Geometry check sheet. Reference: drawing and pictorial views, mm from the part's lowest x, y, z. A direction names the side the tool comes from. Round coordinates to 2 decimals unless told otherwise and drop trailing zeros. Write each loop counter-clockwise with the first axis right and the second up, starting at its lowest first coordinate (ties: lowest second). Pieces come first, ordered by that corner, then holes. Notation, with made-up numbers: M -11.75,57.25 L 13.25,57.25 A25 ccw 13.25,92.25 Z; hole C 28,-6 d10. An arc over 180 degrees is marked long. Answer in a Markdown table with one row per item.
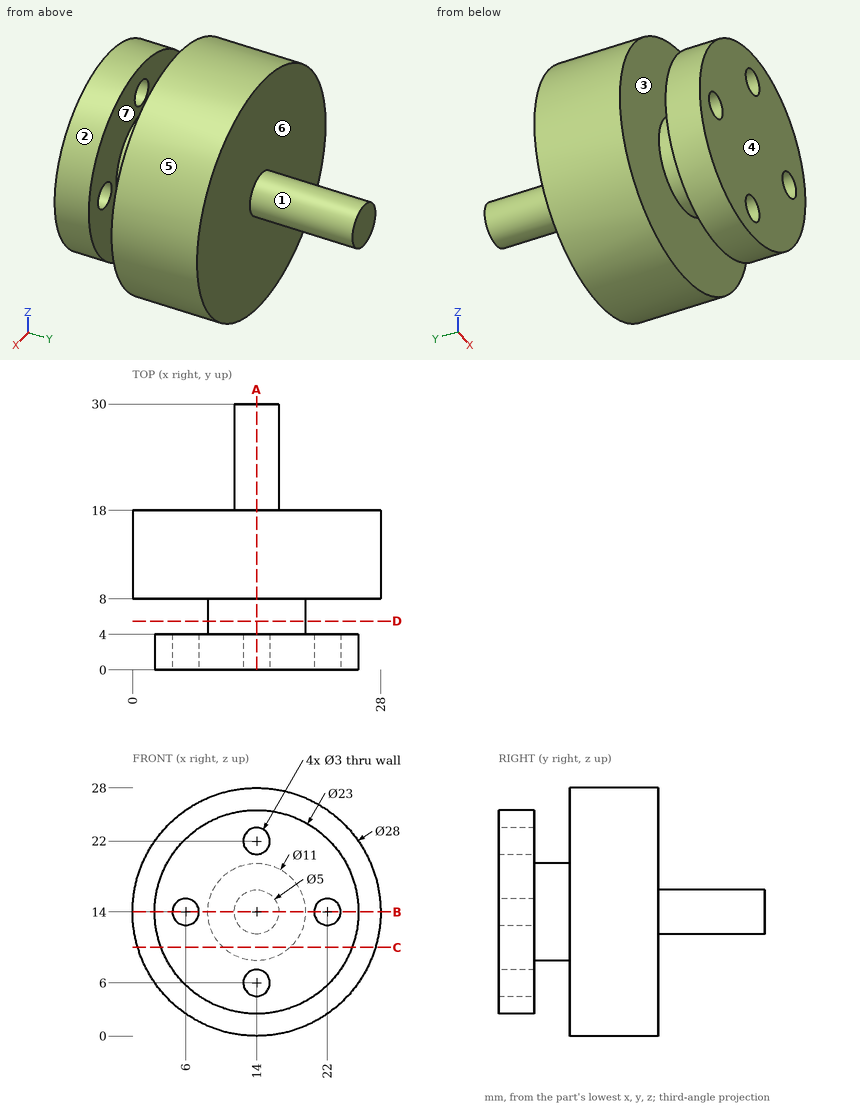
1. Section check C-C, the plane z = 10. Record the cut outline in (x, y).
Found:
| item | result |
|---|---|
| outline | M 0.58,8 L 10.23,8 L 10.23,4 L 3.22,4 L 3.22,0 L 24.78,0 L 24.78,4 L 17.77,4 L 17.77,8 L 27.42,8 L 27.42,18 L 0.58,18 Z |
2. Scan lines: L1, parallel to X at y = 3, z = 14; L2, parallel to Y at x = 8.5, z = 23; L3, parallel to Y at x = 18.5, z = 25.5. Record each from-to range of solid material in increasing order.
Found:
| item | result |
|---|---|
| L1 | x = 2.5 to 4.5, 7.5 to 20.5, 23.5 to 25.5 |
| L2 | y = 0 to 4, 8 to 18 |
| L3 | y = 8 to 18 |
3. Draft check along Y on the marked faces 4, 5, 6 and 7. Enter one of: +Y half, -Y half, draft (parallel to the pull), parting line (faces both ways), or undercut.
Found:
| item | result |
|---|---|
| face 4 | -Y half |
| face 5 | draft |
| face 6 | +Y half |
| face 7 | undercut |
4. Go/stop test with flat-tipped pins: pin 1 (3 mm diameter, centred on y = 5, z = 10, fed in from -X); pin 2 (3 mm diameter, centred on x = 7.5, y = 3.5, fed in from +Z); pin 3 (1.8 mm diameter, centred on x = 6, z = 14, fed in from +Y); pin 4 (1 mm diameter, centred on x = 4, y = 19, fed in from +Z). Record where each tip stops, or that it passes through.
Found:
| item | result |
|---|---|
| pin 1 | stops at x = 2.87 |
| pin 2 | stops at z = 24.36 |
| pin 3 | stops at y = 18 |
| pin 4 | passes through |
5. Section check A-A, the plane x = 14. Record the cut outline in (y, z).
Found:
| item | result |
|---|---|
| outline | M 0,2.5 L 4,2.5 L 4,4.5 L 0,4.5 Z; M 0,7.5 L 4,7.5 L 4,8.5 L 8,8.5 L 8,0 L 18,0 L 18,11.5 L 30,11.5 L 30,16.5 L 18,16.5 L 18,28 L 8,28 L 8,19.5 L 4,19.5 L 4,20.5 L 0,20.5 Z; M 0,23.5 L 4,23.5 L 4,25.5 L 0,25.5 Z |
6. Section check B-B, the plane z = 14. Record the cut outline in (x, y), and give its area (3 significant figures).
Found:
| item | result |
|---|---|
| outline | M 0,8 L 8.5,8 L 8.5,4 L 7.5,4 L 7.5,0 L 20.5,0 L 20.5,4 L 19.5,4 L 19.5,8 L 28,8 L 28,18 L 16.5,18 L 16.5,30 L 11.5,30 L 11.5,18 L 0,18 Z; M 2.5,0 L 4.5,0 L 4.5,4 L 2.5,4 Z; M 23.5,0 L 25.5,0 L 25.5,4 L 23.5,4 Z |
| area | 452 mm2 |
7. Access from +Z, -Z, +X, -X, +Y, -Y to the whole of each face (thin tool, end or side, straight path). Record for the marked faces 1, 2 and 3.
Found:
| item | result |
|---|---|
| face 1 | +Y |
| face 2 | -Y |
| face 3 | none |
8. Section check D-D, the plane y = 5.5. Record the cut outline in (x, z), and give its area (3 significant figures).
Found:
| item | result |
|---|---|
| outline | C 14,14 d11 |
| area | 95.0 mm2 |
